```python
from build123d import *

# Parameters (mm, degrees)
SKETCH1_R           = 4
BOSS_EXTRUDE1_DEPTH = 50
SKETCH3_R           = 10
BOSS_EXTRUDE2_DEPTH = 5
FILLET1_R           = 2.5
BOSS_EXTRUDE3_DEPTH = 5


with BuildPart() as part:
    # Sketch1 → Boss-Extrude1 (new body)
    with BuildSketch(Plane(origin=(0, 0, 0), x_dir=(1, 0, 0), z_dir=(0, 1, 0))):
        with Locations(Location((0, 0, 0), (0, 0, 270))):
            Circle(SKETCH1_R)
    extrude(amount=BOSS_EXTRUDE1_DEPTH)

    # Sketch3 → Boss-Extrude2 (add)
    with BuildSketch(Plane.XZ):
        with Locations(Location((0, 0, 0), (0, 0, 270))):
            Circle(SKETCH3_R)
    extrude(amount=BOSS_EXTRUDE2_DEPTH)

    # Fillet1
    fillet1_edges = [part.edges().sort_by_distance(p)[0] for p in [
        (0, -5, 10),
    ]]
    fillet(fillet1_edges, radius=FILLET1_R)

    # Sketch4 → Boss-Extrude3 (add, symmetric)
    with BuildSketch(Plane(origin=(0, 0, 0), x_dir=(0, 0, -1), z_dir=(1, 0, 0))):
        with BuildLine():
            Line((-6, -5), (6, -5))
            ThreePointArc((6, -5), (0, -11), (-6, -5))
        make_face()
    extrude(amount=BOSS_EXTRUDE3_DEPTH, both=True)


solid = part.part
```
For this review, take the finished solid that the model builds, in its own axes (mm). A direction names the side the tool comes from. Give positions to 0.01 mm unless a question says otherwise; leave off trailing zeros. Order: outer loops, then holes, each group sorted by start corner. A loop starts at its lowest first (then second) coordinate and runs counter-clockwise, first axis right, second up.
1) Take a section at B-B (x = 0). Give the boundary of the cut face in (y, z), then the cut area to 3 significant figures.
2) For faces 1 (the face through (0, -5, 7)), 2 (the face through (0, -5, -7)), 3 (the face through (-3.905, 24.65, -0.867)), 4 (the face through (5, -7, 0)), 5 (the face through (-6, -5, 0)), list the 3-axis set-ups (+Z, -Z, +X, -X, +Y, -Y) from which the entire face can be reached by the end or side of a thin tool; tool diameter is ignored.
3) Insertion check: pin 1 (6 mm diameter, centred on x = 5, z = 6.5, fed in from +Y); pin 2 (5 mm diameter, centred on x = 4.5, z = -5, fed in from -Y); pin 3 (1.3 mm diameter, centred on x = -6, z = -2.5, fed in from -Y). Each pin has a flat end and moves straight along its axis. Give the tip position at first contact, or say it passes through.
4) Take a section at A-A (z = 0). Give the boundary of the cut face in (x, y).
5) Take a section at C-C (y = 6.5). Give the boundary of the cut face in (x, z), then the cut area to 3 significant figures.
6) Wall thickness on line 1 (Y direction, x = 0.75, z = 7.25); line 2 (X direction, y = 26.5, z = -0.25); line 3 (Y direction, x = -4.25, z = 7): over which ranges is each line inside the solid? List them lowest first.
Derived:
1. outline: (-5, -7.5) arc R2.5 ccw to (-2.5, -10) - (0, -10) - (0, -4) - (50, -4) - (50, 4) - (0, 4) - (0, 10) - (-2.5, 10) arc R2.5 ccw to (-5, 7.5) - (-5, 6) arc R6 ccw to (-5, -6) - close
1. area: 554 mm2
2. face 1: +Z, +X, -X, -Y
2. face 2: -Z, +X, -X, -Y
2. face 3: +Y
2. face 4: +Z, -Z, +X, -Y
2. face 5: +Z, -Z, -X, -Y
3. pin 1: stops at y = 0
3. pin 2: stops at y = -10.45
3. pin 3: stops at y = -5
4. outline: (-10, -2.5) arc R2.5 ccw to (-7.5, -5) - (-5, -5) - (-5, -11) - (5, -11) - (5, -5) - (7.5, -5) arc R2.5 ccw to (10, -2.5) - (10, 0) - (4, 0) - (4, 50) - (-4, 50) - (-4, 0) - (-10, 0) - close
5. outline: circle Ø8 at (0, 0)
5. area: 50.3 mm2
6. line 1: y = -5 to 0
6. line 2: x = -3.99 to 3.99
6. line 3: y = -4.9 to 0
